Input: part model. Units: mm. Frame: model coordinates. Face numbers are marked on the shaded views. A direction names the side the tool comes from. Coordinates: 2 decimals unless noted, no trailing zeros. Order: outer loops, then holes, each group sorted by start corner. A loop starts at its lowest first (then second) coordinate and runs counter-clockwise, first axis right, second up. Notation, with made-up numbers: (18, 6.5) -> (42, 6.5) arc R18 cw to (42, 18.5) -> close; hole circle Ø2 at (89.25, -8.5). An arc over 180 degrees is marked (long way). Write each question's results on one line, items separated by ' | '.
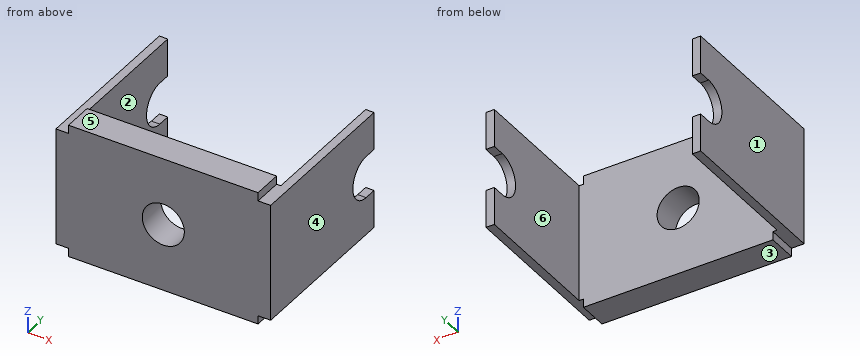
```python
from build123d import *

# Parameters (mm, degrees)
BOSS_EXTRUDE1_DEPTH = 14
BOSS_EXTRUDE2_DEPTH = 22.5
CUT_EXTRUDE1_DEPTH  = 52
SKETCH4_R           = 5
CUT_EXTRUDE2_DEPTH  = 8


with BuildPart() as part:
    # Sketch1 → Boss-Extrude1 (new body, symmetric)
    with BuildSketch(Plane.XY):
        Polygon((-25.5, 3), (-25.5, -36), (25.5, -36), (25.5, 3), (23.5, 3), (23.5, -29), (-23.5, -29), (-23.5, 3), align=None)
    extrude(amount=BOSS_EXTRUDE1_DEPTH, both=True)

    # Sketch2 → Boss-Extrude2 (add, symmetric)
    with BuildSketch(Plane(origin=(0, 0, 0), x_dir=(0, 0, -1), z_dir=(1, 0, 0))):
        Polygon((-14, -36), (-16, -36), (-16, -29), (-13, -29), (-13, -33), (-14, -33), align=None)
    boss_extrude2 = extrude(amount=BOSS_EXTRUDE2_DEPTH, both=True)

    # Mirror1: Boss-Extrude2 across plane
    add(boss_extrude2.mirror(Plane.XY))

    # Sketch3 → Cut-Extrude1 (cut, through all)
    with BuildSketch(Plane(origin=(25.5, 0, 0), x_dir=(0, 0, -1), z_dir=(1, 0, 0))):
        with BuildLine():
            Line((-5, 0), (-5, 3))
            Line((-5, 3), (5, 3))
            Line((5, 3), (5, 0))
            ThreePointArc((5, 0), (0, -5), (-5, 0))
        make_face()
    extrude(amount=-CUT_EXTRUDE1_DEPTH, mode=Mode.SUBTRACT)

    # Sketch4 → Cut-Extrude2 (cut, through all)
    with BuildSketch(Plane(origin=(0, -29, 0), x_dir=(1, 0, 0), z_dir=(0, 1, 0))):
        Circle(SKETCH4_R)
    extrude(amount=-CUT_EXTRUDE2_DEPTH, mode=Mode.SUBTRACT)


solid = part.part
```
(1) Pin query (flat end, axial travel): P1, Ø0.6, axis at y = -32, z = 14.5, coming from the -X side; P2, Ø2.5, axis at x = -23.5, y = -19.5, coming from the -Z side; P3, Ø11.5, axis at x = 0, z = 0, coming from the -Y side; P4, Ø2.5, axis at x = 24, y = -15.5, coming from the +Z side. Return the tip coordinate at first contact, or that it passes through.
Return value:
P1: x = -22.5 | P2: z = -14 | P3: y = -36 | P4: z = 14
(2) Cut plane A-A, the plane z = 0. Return loops of the section in (x, y).
Return value:
outline: (-25.5, -36) -> (-5, -36) -> (-5, -29) -> (-23.5, -29) -> (-23.5, -5) -> (-25.5, -5) -> close; (5, -36) -> (25.5, -36) -> (25.5, -5) -> (23.5, -5) -> (23.5, -29) -> (5, -29) -> close
(3) Mould query, pull axis X, two halves, no side actions, for the marked faces 1, 2, 3 and 4. Classes: +X half, -X half, draft (parallel to the pull), parting line (faces both ways), or undercut.
Return value:
face 1: -X half | face 2: undercut | face 3: draft | face 4: +X half
(4) Cut plane B-B, the plane x = 0. Return loops of the section in (y, z).
Return value:
outline: (-36, -16) -> (-29, -16) -> (-29, -5) -> (-36, -5) -> close; (-36, 5) -> (-29, 5) -> (-29, 16) -> (-36, 16) -> close
(5) Cut plane C-C, the plane y = -17. Return loops of the section in (x, z), plus the area to 3 significant figures.
Return value:
outline: (-25.5, -14) -> (-23.5, -14) -> (-23.5, 14) -> (-25.5, 14) -> close; (23.5, -14) -> (25.5, -14) -> (25.5, 14) -> (23.5, 14) -> close | area: 112 mm2
(6) Line query: line 1 along Z through (x, y) = (0, -33.75); line 2 along X through (y, z) = (-12, 3); line 3 along X through (y, z) = (-33, 0). Output: solid intervals per line, ascending. Write a range as from..to.
Return value:
line 1: -16..-5, 5..16 | line 2: -25.5..-23.5, 23.5..25.5 | line 3: -25.5..-5, 5..25.5
(7) Cut plane D-D, the plane z = 13. Return loops of the section in (x, y).
Return value:
outline: (-25.5, -36) -> (25.5, -36) -> (25.5, 3) -> (23.5, 3) -> (23.5, -29) -> (-23.5, -29) -> (-23.5, 3) -> (-25.5, 3) -> close
(8) Reachability of the marked faces 5 and 6 from +Z, -Z, +X, -X, +Y, -Y: full face, straight path, thin tool, end or side. Return the list, or none.
Return value:
face 5: +Z, +X, -X, +Y, -Y | face 6: +Z, -Z, +Y
